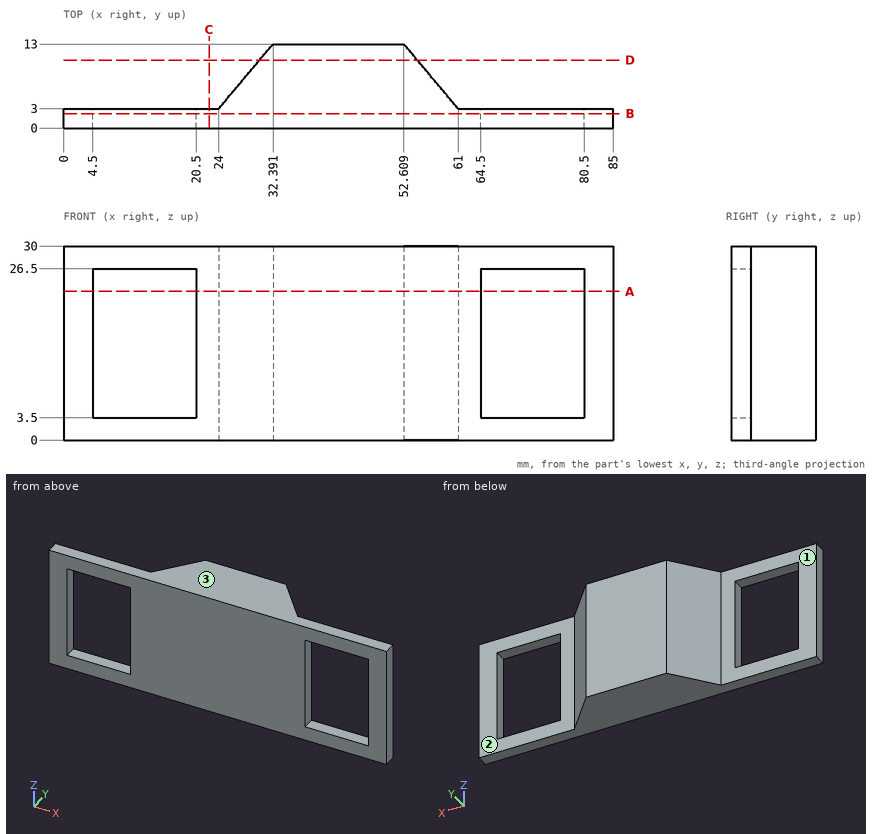
Verification items for this drawing (mm, ordinates from the low corner). A direction names the side the tool comes from. Give positions to 0.01 mm unless a question says otherwise; leave off trailing zeros. Loops run counter-clockwise (first coordinate to the right, second up) from the corner with the lowest first, then second, coordinate; pieces in that order, holes last. Notation, with made-up numbers: M 62,21 L 90,21 A32 cw 90,51 Z; hole C -26,-39 d9. An arc over 180 degrees is marked long. Answer as a JSON object with one key per item and string values. Group by question number.
Q1. Material ranges on line 1 along X through (y, z) = (1, 24); line 2 along Z through (x, y) = (79.5, 2.75); line 3 along Y through (x, z) = (63, 26), recorded low to high. Write a range as [from, to].
Q2. Access from +Z, -Z, +X, -X, +Y, -Y to the whole of each face (thin tool, end or side, straight path). Record for the marked faces 1, 2 and 3.
Q3. Go/stop test with flat-tipped pins: P1, Ø1.5, axis at y = 6, z = 24, coming from the -X side; P2, Ø5, axis at y = 8.5, z = 24.5, coming from the +X side; P3, Ø7, axis at x = 7.5, z = 20, coming from the +Y side. Record where each tip stops, or that it passes through.
Q4. Cross-section at A-A on z = 23. Give the number of separate pieces and of enclosed holes in the cut face, then the cut area to 3 significant figures.
Q5. Cross-section at B-B on y = 2.25. Record the cut outline in (x, z).
Q6. Cross-section at C-C on x = 22.5. Record the cut outline in (y, z).
Q7. Cross-section at D-D on y = 10.5. Record the cut outline in (x, z), then the cut area to 3 significant figures.
Evaluation:
{
 "1": {"line 1": "x = [0, 4.5], [20.5, 64.5], [80.5, 85]", "line 2": "z = [0, 3.5], [26.5, 30]", "line 3": "y = [0, 3]"},
 "2": {"face 1": "+Z, -Z, -X, +Y", "face 2": "+Z, -Z, +X, +Y", "face 3": "+Z, +X, -X, +Y, -Y"},
 "3": {"P1": "stops at x = 25.89", "P2": "stops at x = 58.48", "P3": "stops at y = 3"},
 "4": {"separate pieces": "3", "enclosed holes": "0", "area": "445 mm2"},
 "5": {"outline": "M 0,0 L 85,0 L 85,30 L 0,30 Z; hole M 4.5,3.5 L 20.5,3.5 L 20.5,26.5 L 4.5,26.5 Z; hole M 64.5,3.5 L 80.5,3.5 L 80.5,26.5 L 64.5,26.5 Z"},
 "6": {"outline": "M 0,0 L 3,0 L 3,30 L 0,30 Z"},
 "7": {"outline": "M 30.29,0 L 54.71,0 L 54.71,30 L 30.29,30 Z", "area": "732 mm2"}
}
